```python
from build123d import *

# Parameters (mm, degrees)
BOSS_EXTRUDE1_DEPTH = 8
SKETCH2_OUTSIDE_W   = 41.62
SKETCH2_OUTSIDE_H   = 39.144
SKETCH2_OUTSIDE_R   = 8
CUT_EXTRUDE1_DEPTH  = 8
CUT_EXTRUDE1_TAPER  = 45
SKETCH3_R           = 4
BOSS_EXTRUDE2_DEPTH = 25


with BuildPart() as part:
    # Sketch1 → Boss-Extrude1 (new body)
    with BuildSketch(Plane.XY):
        Polygon((9.237604307, 0), (4.618802154, 8), (-4.618802154, 8), (-9.237604307, 0), (-4.618802154, -8), (4.618802154, -8), align=None)
    extrude(amount=BOSS_EXTRUDE1_DEPTH)

    # Sketch2 outside → Cut-Extrude1 (cut)
    with BuildSketch(Plane.XY.offset(8)):
        Rectangle(SKETCH2_OUTSIDE_W, SKETCH2_OUTSIDE_H)
        Circle(SKETCH2_OUTSIDE_R, mode=Mode.SUBTRACT)
    extrude(amount=-CUT_EXTRUDE1_DEPTH, taper=CUT_EXTRUDE1_TAPER, mode=Mode.SUBTRACT)

    # Sketch3 → Boss-Extrude2 (add)
    with BuildSketch(Plane(origin=(0, 0, 0), x_dir=(-1, 0, 0), z_dir=(0, 0, -1))):
        with Locations(Location((0, 0, 0), (0, 0, 180))):  # turned: the seam where the file's is
            Circle(SKETCH3_R)
    extrude(amount=BOSS_EXTRUDE2_DEPTH)


solid = part.part
```
For this review, take the finished solid that the model builds, in its own axes (mm). A direction names the side the tool comes from. Give positions to 0.01 mm unless a question says otherwise; leave off trailing zeros. Write each loop counter-clockwise with the first axis right and the second up, starting at its lowest first coordinate (ties: lowest second). Pieces come first, ordered by that corner, then holes. Notation, with made-up numbers: M 49,21.5 L 75,21.5 A19 cw 75,38.5 Z; hole C 70.25,43 d11. An arc over 180 degrees is marked long. Answer as a JSON object with one key per item and string values. Group by question number.
Item 1: For pin 1 Ø3 at (x, z) = (6, -8.5) entering from +Y; pin 2 Ø8 at (y, z) = (4, -13) entering from +X; pin 3 Ø1.5 at (y, z) = (1, -7.5) entering from -X; pin 4 Ø1 at (x, y) = (-1.5, 6.5) entering from -Z, all flat-tipped, find the tip position at first contact; note any pin that passes through.
Item 2: Tool access review of faces 1 (the conical face through (-8.3, 0, 7.7)), 2 (the cylindrical face through (-0.867, 3.905, -12.325)): name each direction out of +Z, -Z, +X, -X, +Y, -Y from which nothing blocks a thin tool from reaching the whole face with its end or side.
Item 3: Consider section A-A on z = 4.5. Write out the cut boundary in (x, y), plus the area to 3 significant figures.
Item 4: For probe 1 along Z at (x, y) = (5.5, 4.25); probe 2 along X at (y, z) = (-0.25, -10.5); probe 3 along Y at (x, z) = (0, -13), list the stretches that pass through material, from the lowest coordinate up. Write a range as [from, to].
Item 5: Consider section B-B on z = -20.5. Write out the cut boundary in (x, y), plus the area to 3 significant figures.
Check result:
{
 "1": {"pin 1": "passes through", "pin 2": "stops at x = 4", "pin 3": "stops at x = -3.99", "pin 4": "stops at z = 0"},
 "2": {"face 1": "+Z, -X", "face 2": "-Z"},
 "3": {"outline": "M -9.24,0 L -4.62,-8 L 4.62,-8 L 9.24,0 L 4.62,8 L -4.62,8 Z", "area": "222 mm^2"},
 "4": {"probe 1": "z = [0, 8]", "probe 2": "x = [-3.99, 3.99]", "probe 3": "y = [-4, 4]"},
 "5": {"outline": "C 0,0 d8", "area": "50.3 mm^2"}
}
